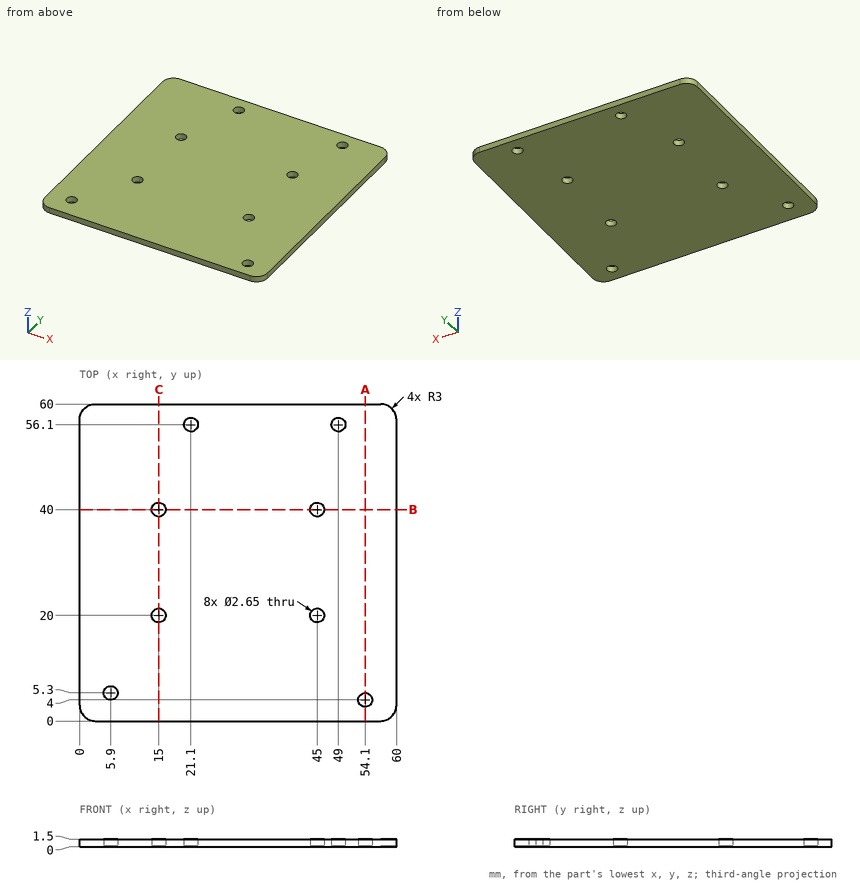
Job drawing, mm, ordinate dimensions from the low corner. One solid piece. Give positions to 0.01 mm unless a question says otherwise; leave off trailing zeros. Order: outer loops, then holes, each group sorted by start corner. A loop starts at its lowest first (then second) coordinate and runs counter-clockwise, first axis right, second up. Notation, with made-up numbers: (-26, 28) - (4, 28) arc R14 cw to (4, 46) - close; hole circle Ø11 at (20, -14.5). An arc over 180 degrees is marked (long way). Return JSON: item names as keys, results as strings.
1) Cut at C-C, the plane x = 15. Give the cut face in (y, z) (3 decimals), plus the area to 4 significant figures.
Geometry says:
{"outline": "(0, 0) - (18.675, 0) - (18.675, 1.5) - (0, 1.5) - close; (21.325, 0) - (38.675, 0) - (38.675, 1.5) - (21.325, 1.5) - close; (41.325, 0) - (60, 0) - (60, 1.5) - (41.325, 1.5) - close", "area": "82.05 mm²"}
2) Cut at B-B, the plane y = 40. Give the cut face in (x, z) (3 decimals), plus the area to 4 significant figures.
Geometry says:
{"outline": "(0, 0) - (13.675, 0) - (13.675, 1.5) - (0, 1.5) - close; (16.325, 0) - (43.675, 0) - (43.675, 1.5) - (16.325, 1.5) - close; (46.325, 0) - (60, 0) - (60, 1.5) - (46.325, 1.5) - close", "area": "82.05 mm²"}
3) Probe line 1 (Y direction, x = 45, z = 0.7) (3 decimals); line 2 (Y direction, x = 21.1, z = 1.1) (3 decimals); line 3 (Y direction, x = 54.1, z = 1.15) (3 decimals). List the from-to ranges inside material, lowest first. Write a range as from..to.
Geometry says:
{"line 1": "0..18.675, 21.325..38.675, 41.325..60", "line 2": "0..54.775, 57.425..60", "line 3": "0..2.675, 5.325..60"}
4) Flat gauge pin, fed straight in: P1, Ø1.6, axis at x = 54.1, y = 4, coming from the +Z side. Where does the tip first touch, or does it go through?
Geometry says:
{"P1": "through"}
5) Cut at A-A, the plane x = 54.1. Give the cut face in (y, z) (3 decimals), plus the area to 3 significant figures.
Geometry says:
{"outline": "(0, 0) - (2.675, 0) - (2.675, 1.5) - (0, 1.5) - close; (5.325, 0) - (60, 0) - (60, 1.5) - (5.325, 1.5) - close", "area": "86.0 mm²"}
